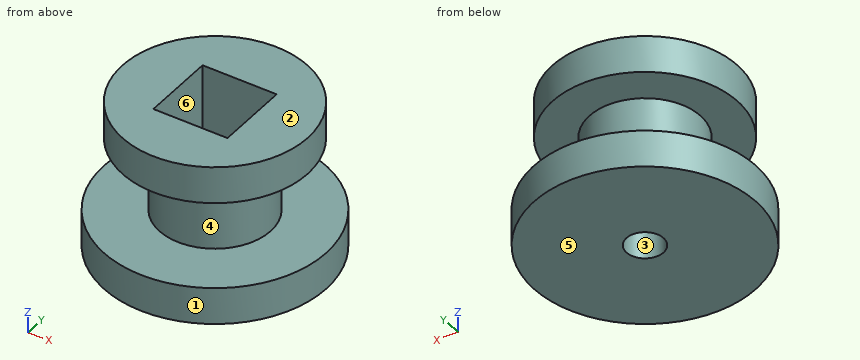
```python
from build123d import *

# Parameters (mm, degrees)
F0_R     = 38.1
F1_DEPTH = 12.7
F2_R     = 19.05
F3_DEPTH = 25.4
F4_R     = 31.75
F5_DEPTH = 12.7
F6_W     = 25.4
F6_H     = 25.4
F7_DEPTH = 25.4
F8_R     = 6.35
F9_DEPTH = 50.801


with BuildPart() as f1:
    # F0 (on Top) → F1 (new body)
    with BuildSketch(Plane.XY):
        Circle(F0_R)
    extrude(amount=F1_DEPTH)

    # F2 (on face) → F3 (join)
    with BuildSketch(Plane.XY.offset(12.7)):
        Circle(F2_R)
    extrude(amount=F3_DEPTH)

    # F4 (on face) → F5 (join)
    with BuildSketch(Plane.XY.offset(38.1)):
        Circle(F4_R)
    extrude(amount=F5_DEPTH)

    # F6 (on face) → F7 (cut)
    with BuildSketch(Plane.XY.offset(50.8)):
        Rectangle(F6_W, F6_H)
    extrude(amount=-F7_DEPTH, mode=Mode.SUBTRACT)

    # F8 (on face) → F9 (cut, through all)
    with BuildSketch(Plane.XY.offset(50.8)):
        Circle(F8_R)
    extrude(amount=-F9_DEPTH, mode=Mode.SUBTRACT)


solid = f1.part
```
CAD build for the part. Positions are in the model's coordinates, mm. Face numbers are marked on the shaded views. A direction names the side the tool comes from. Round coordinates to 2 decimals unless told otherwise and drop trailing zeros. Loops run counter-clockwise (first coordinate to the right, second up) from the corner with the lowest first, then second, coordinate; pieces in that order, holes last. Notation, with made-up numbers: (31, 39.5) - (73, 39.5) arc R16 ccw to (73, 47.5) - close; hole circle Ø11 at (49.25, 79). An arc over 180 degrees is marked (long way). Return JSON: item names as keys, results as strings. Group by question number.
Q1. Band-saw the part on C-C on z = 41.5. Give the cut face in (x, y), plus the area to 3 significant figures.
Q2. Tool access for the marked faces 4, 5 and 6: list every direction of +Z, -Z, +X, -X, +Y, -Y with a clear straight run to the whole face (end or side of a thin tool).
Q3. Two-plate mould, pull along Y, no slides. Class the marked faces 1, 2 and 3: +Y half, -Y half, draft (parallel to the pull), parting line (faces both ways), or undercut.
Q4. Drill centre lines: line 1 along Z through (x, y) = (20, 24); line 2 along Y through (x, z) = (0, 13.75); line 3 along Y through (x, z) = (0, 8). Where is each one in solid material? Low to high. Write a range as [from, to].
Q5. Band-saw the part on D-D on y = -10.5. Give the cut face in (x, z), plus the area to 3 significant figures.
Q6. Band-saw the part on A-A on x = 0. Give the cut face in (y, z).
Q7. Flat gauge pins, fed straight in: pin 1 Ø12 at (y, z) = (-3.5, 19) entering from +X; pin 2 Ø6 at (y, z) = (11.5, 33) entering from -X; pin 3 Ø7.5 at (y, z) = (-3.5, 34.5) entering from -X. Where does each tip first touch, or does it go through?
Solutions:
{
 "1": {"outline": "circle Ø63.5 at (0, 0); hole (-12.7, -12.7) - (12.7, -12.7) - (12.7, 12.7) - (-12.7, 12.7) - close", "area": "2,520 mm^2"},
 "2": {"face 4": "none", "face 5": "-Z, +X, -X, +Y, -Y", "face 6": "+Z"},
 "3": {"face 1": "parting line", "face 2": "draft", "face 3": "undercut"},
 "4": {"line 1": "z = [0, 12.7], [38.1, 50.8]", "line 2": "y = [-19.05, -6.35], [6.35, 19.05]", "line 3": "y = [-38.1, -6.35], [6.35, 38.1]"},
 "5": {"outline": "(-36.62, 0) - (36.62, 0) - (36.62, 12.7) - (15.9, 12.7) - (15.9, 38.1) - (29.96, 38.1) - (29.96, 50.8) - (12.7, 50.8) - (12.7, 25.4) - (-12.7, 25.4) - (-12.7, 50.8) - (-29.96, 50.8) - (-29.96, 38.1) - (-15.9, 38.1) - (-15.9, 12.7) - (-36.62, 12.7) - close", "area": "1,850 mm^2"},
 "6": {"outline": "(-38.1, 0) - (-6.35, 0) - (-6.35, 25.4) - (-12.7, 25.4) - (-12.7, 50.8) - (-31.75, 50.8) - (-31.75, 38.1) - (-19.05, 38.1) - (-19.05, 12.7) - (-38.1, 12.7) - close; (6.35, 0) - (38.1, 0) - (38.1, 12.7) - (19.05, 12.7) - (19.05, 38.1) - (31.75, 38.1) - (31.75, 50.8) - (12.7, 50.8) - (12.7, 25.4) - (6.35, 25.4) - close"},
 "7": {"pin 1": "stops at x = 19.05", "pin 2": "stops at x = -17.05", "pin 3": "stops at x = -31.66"}
}
